Check sheet for the modelled part. Datum: model origin and axes. Units: mm. Round coordinates to 2 decimals unless told otherwise and drop trailing zeros. Write each loop counter-clockwise with the first axis right and the second up, starting at its lowest first coordinate (ties: lowest second). Pieces come first, ordered by that corner, then holes. Notation, with made-up numbers: M -20,47 L 22,47 A18 ccw 22,61 Z; hole C 81.25,1 d11. An arc over 180 degrees is marked long. Put each result on its own line as item: value.
```python
from build123d import *

# Parameters (mm, degrees)
F0_W     = 50.8
F0_H     = 57.4548
F1_DEPTH = 6.35
F2_D     = 4.4958
F3_D     = 4.4958
F4_D     = 4.4958
F5_D     = 4.4958
F6_D     = 4.4958
F7_D     = 4.4958
F8_D     = 4.4958


with BuildPart() as f1:
    # F0 (on Top) → F1 (new body)
    with BuildSketch(Plane.XY):
        Rectangle(F0_W, F0_H)
    extrude(amount=F1_DEPTH)

    # F2 (through all)
    with Locations(Plane(origin=(0, 0, 0), x_dir=(1, 0, 0), z_dir=(0, 0, -1))):
        with Locations((-20.32, 13.4747)):
            Hole(F2_D / 2)

    # F3 (through all)
    with Locations(Plane(origin=(0, 0, 0), x_dir=(1, 0, 0), z_dir=(0, 0, -1))):
        with Locations((-20.32, -13.4747)):
            Hole(F3_D / 2)

    # F4 (through all)
    with Locations(Plane(origin=(0, 0, 0), x_dir=(1, 0, 0), z_dir=(0, 0, -1))):
        with Locations((6.6294, -13.4747)):
            Hole(F4_D / 2)

    # F5 (through all)
    with Locations(Plane(origin=(0, 0, 0), x_dir=(1, 0, 0), z_dir=(0, 0, -1))):
        with Locations((6.6294, 13.4747)):
            Hole(F5_D / 2)

    # F6 (through all)
    with Locations(Plane(origin=(0, 0, 0), x_dir=(1, 0, 0), z_dir=(0, 0, -1))):
        with Locations((20.32, 23.6474)):
            Hole(F6_D / 2)

    # F7 (through all)
    with Locations(Plane(origin=(0, 0, 0), x_dir=(1, 0, 0), z_dir=(0, 0, -1))):
        with Locations((20.32, 0)):
            Hole(F7_D / 2)

    # F8 (through all)
    with Locations(Plane(origin=(0, 0, 0), x_dir=(1, 0, 0), z_dir=(0, 0, -1))):
        with Locations((20.32, -23.6474)):
            Hole(F8_D / 2)


solid = f1.part
```
1. Depth check by flat-ended pin: pin 1 Ø7 at (x, y) = (6.63, -13.47) entering from -Z. Enter the tip coordinate at first touch or a pass-through.
Computed values:
pin 1: stops at z = 0
2. Cross-section at D-D (z = 1.25). Enter the section's corners in (x, y).
Computed values:
outline: M -25.4,-28.73 L 25.4,-28.73 L 25.4,28.73 L -25.4,28.73 Z; hole C -20.32,-13.47 d4.5; hole C -20.32,13.47 d4.5; hole C 6.63,-13.47 d4.5; hole C 6.63,13.47 d4.5; hole C 20.32,-23.65 d4.5; hole C 20.32,0 d4.5; hole C 20.32,23.65 d4.5
3. Cross-section at B-B (x = -20.32). Enter the section's corners in (y, z).
Computed values:
outline: M -28.73,0 L -15.72,0 L -15.72,6.35 L -28.73,6.35 Z; M -11.23,0 L 11.23,0 L 11.23,6.35 L -11.23,6.35 Z; M 15.72,0 L 28.73,0 L 28.73,6.35 L 15.72,6.35 Z
4. Cross-section at C-C (x = 20.32). Enter the section's corners in (y, z), then the cut area to 3 significant figures.
Computed values:
outline: M -28.73,0 L -25.9,0 L -25.9,6.35 L -28.73,6.35 Z; M -21.4,0 L -2.25,0 L -2.25,6.35 L -21.4,6.35 Z; M 2.25,0 L 21.4,0 L 21.4,6.35 L 2.25,6.35 Z; M 25.9,0 L 28.73,0 L 28.73,6.35 L 25.9,6.35 Z
area: 279 mm2
5. Release check for a two-part mould opening along X. For faces 1 (the cylindrical face through (-18.66, 11.96, 3.22)), 2 (the flat face through (0, 28.727, 3)), 3 (the flat face through (25.4, 0, 3)) record: +X half, -X half, draft (parallel to the pull), parting line (faces both ways), or undercut.
Computed values:
face 1: undercut
face 2: draft
face 3: +X half
6. Scan lines: probe 1 along Y at (x, z) = (20.32, 4.5); probe 2 along X at (y, z) = (13.5, 2.5); probe 3 along Y at (x, z) = (-20.32, 3). Record each from-to range of solid material in increasing order.
Computed values:
probe 1: y = -28.73 to -25.9, -21.4 to -2.25, 2.25 to 21.4, 25.9 to 28.73
probe 2: x = -25.4 to -22.57, -18.07 to 4.38, 8.88 to 25.4
probe 3: y = -28.73 to -15.72, -11.23 to 11.23, 15.72 to 28.73
7. Cross-section at A-A (y = 0). Enter the section's corners in (x, z).
Computed values:
outline: M -25.4,0 L 18.07,0 L 18.07,6.35 L -25.4,6.35 Z; M 22.57,0 L 25.4,0 L 25.4,6.35 L 22.57,6.35 Z
